Autodesk Inventor part; units mm, degrees
ref_plane "YZ Plane" through (0, 0, 0) normal (1, 0, 0) x (0, 1, 0)
ref_plane "XZ Plane" through (0, 0, 0) normal (0, 1, 0) x (-1, 0, 0)
ref_plane "XY Plane" through (0, 0, 0) normal (0, 0, 1) x (1, 0, 0)
sketch "Sketch1" plane through (0, 0, 0) normal (0, 1, 0) x (-1, 0, 0)
  circle A0 centre (0, 0) radius 53.125
  circle A1 centre (0, 0) radius 37.5
  dimension "d0" = 106.25
  dimension "d1" = 75
extrude "Extrusion1" add sketch "Sketch1" along normal blind 15
sketch "Sketch2" plane through (0, 0, 0) normal (0, -1, 0) x (1, 0, 0)
  circle A0 centre (0, 0) radius 41.25
  circle A1 centre (-41.25, 0) radius 2.5
  circle A2 centre (-29.1682, -29.1682) radius 2.5
  circle A3 centre (0, -41.25) radius 2.5
  circle A4 centre (29.1682, -29.1682) radius 2.5
  circle A5 centre (41.25, 0) radius 2.5
  circle A6 centre (29.1682, 29.1682) radius 2.5
  circle A7 centre (0, 41.25) radius 2.5
  circle A8 centre (-29.1682, 29.1682) radius 2.5
  dimension "d4" = 82.5
  dimension "d5" = 5
  dimension "d8" = 360
extrude "Extrusion2" cut sketch "Sketch2" against normal blind 3 contours A0 A5 | A0 A5 | A6 A0 | A0 A6 | A4 A0 | A0 A4 | A7 A0 | A0 A7 | A3 A0 | A0 A3 | A8 A0 | A0 A8 | A2 A0 | A0 A2 | A1 A0 | A0 A1
sketch "Sketch3" plane through (0, 15, 0) normal (0, 1, 0) x (1, 0, 0)
  circle A0 centre (0, 0) radius 45.5
  circle A1 centre (45.5, 0) radius 3.5
  circle A2 centre (32.1734, 32.1734) radius 3.5
  circle A3 centre (0, 45.5) radius 3.5
  circle A4 centre (-32.1734, 32.1734) radius 3.5
  circle A5 centre (-45.5, 0) radius 3.5
  circle A6 centre (-32.1734, -32.1734) radius 3.5
  circle A7 centre (0, -45.5) radius 3.5
  circle A8 centre (32.1734, -32.1734) radius 3.5
  dimension "d12" = 91
  dimension "d13" = 7
  dimension "d16" = 360
extrude "Extrusion3" cut sketch "Sketch3" against normal blind 7 contours A0 A1 | A0 A1 | A2 A0 | A0 A2 | A8 A0 | A0 A8 | A3 A0 | A0 A3 | A7 A0 | A0 A7 | A4 A0 | A0 A4 | A6 A0 | A0 A6 | A5 A0 | A0 A5
properties part number "Magnet Spacer"
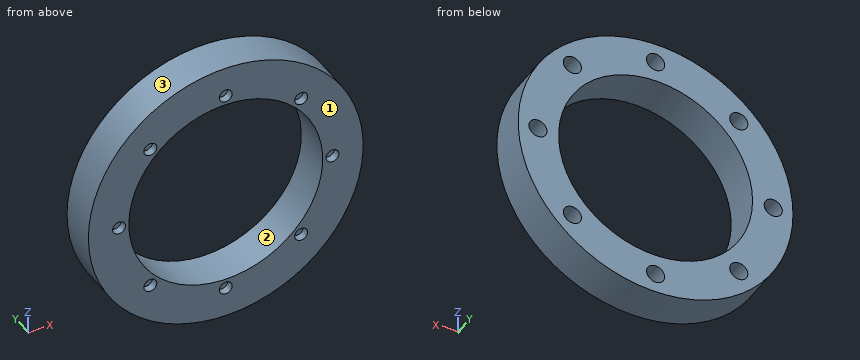
Geometry: final body of the model. Coordinates: model frame, mm. Face numbers are marked on the shaded views. Round coordinates to 2 decimals unless told otherwise and drop trailing zeros. Loops run counter-clockwise (first coordinate to the right, second up) from the corner with the lowest first, then second, coordinate; pieces in that order, holes last. Notation, with made-up numbers: (-39, 72) -> (5, 72) arc R22 ccw to (5, 84) -> close; hole circle Ø6 at (74, -32). An arc over 180 degrees is marked (long way). Use one line per item in the form item = value. Start each with the question number.
1) Section C-C on y = 4.5. Output: boundary loops of the cut face in (x, z) (3 decimals), then the cut area to 3 significant figures.
2) Section B-B on x = 34. Output: boundary loops of the cut face in (y, z).
3) Section A-A on z = 0. Output: boundary loops of the cut face in (x, y) (3 decimals), then the cut area to 3 significant figures.
4) Section D-D on y = 11.5. Give the number of separate pieces and of enclosed holes in the cut face, then the cut area to 3 significant figures.
5) Draft query along Z for the marked faces 1, 2 and 3. Return one class per face: released by +Z, released by -Z, zero draft, split by the parting line, or undercut.
6) First-contact query: P1, Ø7.5, axis at x = 33, z = -33.5, coming from the +Y side; P2, Ø6, axis at y = 5, z = 39.5, coming from the -X side; P3, Ø2, axis at x = -33.5, z = 31, coming from the +Y side; P4, Ø5, axis at y = 7.5, z = -9, coming from the +X side. Flat tips, straight axial feed; report the tip coordinate or a pass-through.
7) Line query: L1, parallel to Z at x = 0, y = 6.25 (3 decimals); L2, parallel to Z at x = -33, y = 11.5; L3, parallel to Z at x = -2, y = 10. Output: solid intervals per line, ascending.
Response:
q1.outline = circle Ø106.25 at (0, 0); hole circle Ø75 at (0, 0)
q1.area = 4,450 mm^2
q2.outline = (0, -40.82) -> (15, -40.82) -> (15, -35.16) -> (8, -35.16) -> (8, -29.19) -> (15, -29.19) -> (15, -15.82) -> (0, -15.82) -> close; (0, 15.82) -> (15, 15.82) -> (15, 29.19) -> (8, 29.19) -> (8, 35.16) -> (15, 35.16) -> (15, 40.82) -> (0, 40.82) -> close
q3.outline = (-53.125, 0) -> (-43.75, 0) -> (-43.75, 3) -> (-38.75, 3) -> (-38.75, 0) -> (-37.5, 0) -> (-37.5, 15) -> (-42, 15) -> (-42, 8) -> (-49, 8) -> (-49, 15) -> (-53.125, 15) -> close; (37.5, 0) -> (38.75, 0) -> (38.75, 3) -> (43.75, 3) -> (43.75, 0) -> (53.125, 0) -> (53.125, 15) -> (49, 15) -> (49, 8) -> (42, 8) -> (42, 15) -> (37.5, 15) -> close
q3.area = 341 mm^2
q4.separate_pieces = 1
q4.enclosed_holes = 9
q4.area = 4,140 mm^2
q5.face_1 = zero draft
q5.face_2 = undercut
q5.face_3 = split by the parting line
q6.P1 = 15
q6.P2 = -38.6
q6.P3 = 8
q6.P4 = 52.73
q7.L1 = -53.125 to -37.5, 37.5 to 53.125
q7.L2 = -41.63 to -35.57, -28.77 to -17.81, 17.81 to 28.77, 35.57 to 41.63
q7.L3 = -53.09 to -48.37, -42.63 to -37.45, 37.45 to 42.63, 48.37 to 53.09
